from build123d import *

# Parameters (mm, degrees)
BOSS_EXTRUDE2_DEPTH = 60
SKETCH4_R           = 10
BOSS_EXTRUDE3_DEPTH = 75
BOSS_EXTRUDE4_START = 75
SKETCH5_R           = 10
BOSS_EXTRUDE4_DEPTH = 75


with BuildPart() as part:
    # Sketch3 → Boss-Extrude2 (new body)
    with BuildSketch(Plane(origin=(0, 0, 0), x_dir=(1, 0, 0), z_dir=(0, 1, 0))):
        with BuildLine():
            Line((-200, 250), (200, 250))
            ThreePointArc((200, 250), (450, 0), (200, -250))
            Line((200, -250), (-200, -250))
            ThreePointArc((-200, -250), (-450, 0), (-200, 250))
        make_face()
    extrude(amount=BOSS_EXTRUDE2_DEPTH)

    # Sketch4 → Boss-Extrude3 (add)
    with BuildSketch(Plane.XY.offset(250)):
        with Locations(Location((-200, 30, 0), (0, 0, 270))):
            Circle(SKETCH4_R)
        with Locations(Location((200, 30, 0), (0, 0, 270))):
            Circle(SKETCH4_R)
    extrude(amount=BOSS_EXTRUDE3_DEPTH)

    # Sketch5 → Boss-Extrude4 (add)
    with BuildSketch(Plane(origin=(0, 0, -250), x_dir=(-1, 0, 0), z_dir=(0, 0, -1)).offset(BOSS_EXTRUDE4_START)):
        with Locations(Location((-200, 30, 0), (0, 0, 270))):
            Circle(SKETCH5_R)
        with Locations(Location((200, 30, 0), (0, 0, 270))):
            Circle(SKETCH5_R)
    extrude(amount=-BOSS_EXTRUDE4_DEPTH)


solid = part.part
Input: part model. Units: mm. Frame: model coordinates. A direction names the side the tool comes from. Give positions to 0.01 mm unless a question says otherwise; leave off trailing zeros. Write each loop counter-clockwise with the first axis right and the second up, starting at its lowest first coordinate (ties: lowest second). Pieces come first, ordered by that corner, then holes.
Q1. Section A-A, the plane y = 30. Output: boundary loops of the cut face in (x, z).
Q2. Section B-B, the plane x = 59. Output: boundary loops of the cut face in (y, z), plus the area to 3 significant figures.
Q3. Section C-C, the plane z = 137. Output: boundary loops of the cut face in (x, y).
Q4. Pull-direction query (X, two-part tool) for faces 4 (the face through (6, 60, -4)), 5 (the face through (-3, 30, -250)); classes: pulls with the +X half, pulls with the -X half, needs draft (parallel to the pull), parting line crosses it, or undercut.
Q5. First-contact query: P1, Ø10, axis at y = 39.5, z = 123.5, coming from the -X side; P2, Ø2, axis at x = -84.5, y = 18.5, coming from the +Z side; P3, Ø8, axis at x = -311, y = 8.5, coming from the -Z side. Flat tips, straight axial feed; report the tip coordinate or a pass-through.
Q6. Material intervals for probe 1 along Z at (x, y) = (121.5, 37); probe 2 along Z at (x, y) = (203.5, 11), sorted ascending.
Q7. Set-up query: faces 1 (the face through (190.24, 32.17, 286.98)), 2 (the face through (-200, 30, 325)), 3 (the face through (-190.24, 32.17, -288.02)). Return all of +Z, -Z, +X, -X, +Y, -Y with unobstructed straight access to the full face (end or side cutting, diameter ignored); none if empty.
Filled in:
1. outline: (-210, -325) - (-190, -325) - (-190, -250) - (190, -250) - (190, -325) - (210, -325) - (210, -250) - (200, -250) arc R250 ccw to (200, 250) - (210, 250) - (210, 325) - (190, 325) - (190, 250) - (-190, 250) - (-190, 325) - (-210, 325) - (-210, 250) - (-200, 250) arc R250 ccw to (-200, -250) - (-210, -250) - close
2. outline: (0, -250) - (60, -250) - (60, 250) - (0, 250) - close
2. area: 30,000 mm2
3. outline: (-409.12, 0) - (409.12, 0) - (409.12, 60) - (-409.12, 60) - close
4. face 4: needs draft
4. face 5: undercut
5. P1: stops at x = -420.13
5. P2: stops at z = 250
5. P3: stops at z = -225.94
6. probe 1: z = -250 to 250
6. probe 2: z = -249.98 to 249.98
7. face 1: +Z
7. face 2: +Z, +X, -X, +Y, -Y
7. face 3: -Z
